Read the model definition and answer for the solid it produces. Units are mm, in the model's axes. Face numbers are marked on the shaded views. A direction names the side the tool comes from. Round coordinates to 2 decimals unless told otherwise and drop trailing zeros. Write each loop counter-clockwise with the first axis right and the second up, starting at its lowest first coordinate (ties: lowest second). Pieces come first, ordered by that corner, then holes. Notation, with made-up numbers: M 82.25,-3.75 L 92.25,-3.75 A7 cw 92.25,8.25 Z; hole C -16,54.25 d11. An arc over 180 degrees is marked long. Use one line per item in the form item = value. Start each with the question number.
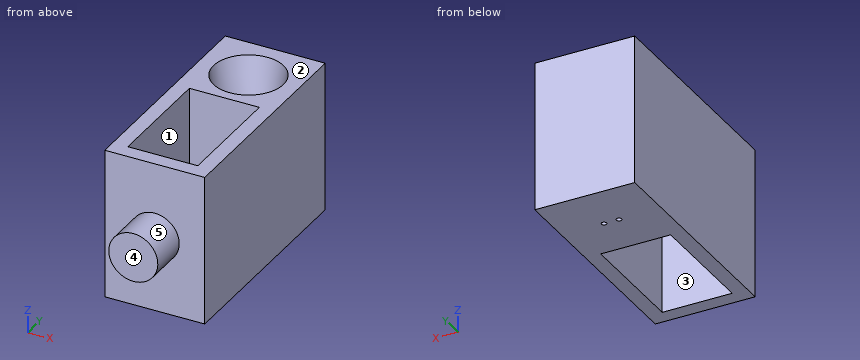
```python
from build123d import *

# Parameters (mm, degrees)
SKETCH1_W           = 20
SKETCH1_H           = 30
BOSS_EXTRUDE1_DEPTH = 45
SKETCH2_R           = 4.9
BOSS_EXTRUDE2_DEPTH = 8
SKETCH3_R           = 7
CUT_EXTRUDE1_DEPTH  = 24
CUT_EXTRUDE1_DRAFT  = -9
SKETCH4_R           = 3.198773432
CUT_EXTRUDE2_DEPTH  = 3
SKETCH5_R           = 0.5
CUT_EXTRUDE3_DEPTH  = 3
SKETCH6_W           = 14
SKETCH6_H           = 23
CUT_EXTRUDE4_DEPTH  = 56


with BuildPart() as part:
    # Sketch1 → Boss-Extrude1 (new body)
    with BuildSketch(Plane(origin=(0, 0, 0), x_dir=(1, 0, 0), z_dir=(0, 1, 0))):
        Rectangle(SKETCH1_W, SKETCH1_H)
    extrude(amount=BOSS_EXTRUDE1_DEPTH)

    # Sketch2 → Boss-Extrude2 (add)
    with BuildSketch(Plane(origin=(0, 0, 0), x_dir=(-1, 0, 0), z_dir=(0, -1, 0))):
        with Locations(Location((0, 0, 0), (0, 0, 90))):
            Circle(SKETCH2_R)
    extrude(amount=BOSS_EXTRUDE2_DEPTH)


with BuildPart() as cut_extrude1_tool:
    # Sketch3 → Cut-Extrude1 (with draft: the straight prism first)
    with BuildSketch(Plane.XY.offset(15)):
        with Locations((0, 35)):
            Circle(SKETCH3_R)
    extrude(amount=-CUT_EXTRUDE1_DEPTH)
    # Cut-Extrude1: the draft: its side faces are tilted about the plane it starts from
    cut_extrude1_sides = [cut_extrude1_tool.faces().sort_by_distance(p)[0] for p in [
        (-7, 35, 3),
    ]]
    draft(cut_extrude1_sides, Plane.XY.offset(15), CUT_EXTRUDE1_DRAFT)


with BuildPart() as part_1:
    add(part.part)

    # Cut-Extrude1: cut by cut_extrude1_tool
    add(cut_extrude1_tool.part, mode=Mode.SUBTRACT)

    # Sketch4 → Cut-Extrude2 (cut)
    with BuildSketch(Plane.XY.offset(-9)):
        with Locations((0, 35)):
            Circle(SKETCH4_R)
    extrude(amount=-CUT_EXTRUDE2_DEPTH, mode=Mode.SUBTRACT)

    # Sketch5 → Cut-Extrude3 (cut)
    with BuildSketch(Plane.XY.offset(-12)):
        with Locations((-1.5, 35)):
            Circle(SKETCH5_R)
        with Locations((1.5, 35)):
            Circle(SKETCH5_R)
    extrude(amount=-CUT_EXTRUDE3_DEPTH, mode=Mode.SUBTRACT)

    # Sketch6 → Cut-Extrude4 (cut, through all)
    with BuildSketch(Plane.XY.offset(15)):
        with Locations((0, 14.5)):
            Rectangle(SKETCH6_W, SKETCH6_H)
    extrude(amount=-CUT_EXTRUDE4_DEPTH, mode=Mode.SUBTRACT)


solid = part_1.part
```
Q1. Find section C-C on z = -2.25. Write down the section's boundary in (x, y).
Q2. Find section A-A on x = 0. Write down the section's boundary in (y, z).
Q3. Find section D-D on x = 7.75. Write down the section's boundary in (y, z).
Q4. For a pull along X with two mould halves and no side action, classify the marked faces 3, 4 and 5 as +X half, -X half, draft (parallel to the pull), parting line (faces both ways), or undercut.
Q5. A tool of negligible diameter and unlimited length cuts with its end or side. For the marked faces 1 and 2, from which of +Z, -Z, +X, -X, +Y, -Y can it reach the whole face along a straight path? Write none if from no direction.
Q6. This flat-tipped pin is pushed along its axis until it touches: pin 1 Ø3 at (x, y) = (-0.5, 33.5) entering from +Z. Where does it stop, or does it pass through?
Q7. Straight lines are drawn through the part: line 1 (Y direction, x = -1.5, z = -14.3); line 2 (X direction, y = 35, z = -13.75); line 3 (Y direction, x = -4.75, z = 7). For each, find the intervals that lie inside material, in ascending order. Write a range as [from, to].
Q8. Find section B-B on y = 12.5. Write down the section's boundary in (x, z), and give its area (3 significant figures).
Response:
q1.outline = M -10,0 L -4.35,0 L -4.35,-8 L 4.35,-8 L 4.35,0 L 10,0 L 10,45 L -10,45 Z; hole M -7,3 L 7,3 L 7,26 L -7,26 Z; hole C 0,35 d8.54
q2.outline = M -8,-4.9 L 0,-4.9 L 0,-15 L 3,-15 L 3,15 L 0,15 L 0,4.9 L -8,4.9 Z; M 26,-15 L 45,-15 L 45,15 L 42,15 L 38.2,-9 L 38.2,-12 L 31.8,-12 L 31.8,-9 L 28,15 L 26,15 Z
q3.outline = M 0,-15 L 45,-15 L 45,15 L 0,15 Z
q4.face_3 = undercut
q4.face_4 = draft
q4.face_5 = parting line
q5.face_1 = +Z, -Z
q5.face_2 = +Z, +X, -X, +Y, -Y
q6.pin_1 = -12
q7.line_1 = [0, 3], [26, 34.5], [35.5, 45]
q7.line_2 = [-10, -2], [-1, 1], [2, 10]
q7.line_3 = [0, 3], [26, 31.79], [38.21, 45]
q8.outline = M -10,-15 L -7,-15 L -7,15 L -10,15 Z; M 7,-15 L 10,-15 L 10,15 L 7,15 Z
q8.area = 180 mm²
